CAD build for the part. Positions are in the model's coordinates, mm. Give positions to 0.01 mm unless a question says otherwise; leave off trailing zeros. Loops run counter-clockwise (first coordinate to the right, second up) from the corner with the lowest first, then second, coordinate; pieces in that order, holes last. Notation, with made-up numbers: M 58.25,18.5 L 106.25,18.5 A23 ccw 106.25,36.5 Z; hole C 50,42.5 d7. An arc over 180 degrees is marked long. Answer as CSV lines item,"result".
Autodesk Inventor part; units mm, degrees
ref_plane "YZ Plane" through (0, 0, 0) normal (1, 0, 0) x (0, 1, 0)
ref_plane "XZ Plane" through (0, 0, 0) normal (0, 1, 0) x (-1, 0, 0)
ref_plane "XY Plane" through (0, 0, 0) normal (0, 0, 1) x (1, 0, 0)
sketch "Sketch1" plane through (0, 0, 0) normal (1, 0, 0) x (0, 1, 0)
  line L0 (0, 0) -> (74.6232, 0)
  line L1 (0, 0) -> (85, -6.078)
  line L2 (85, -6.078) -> (0, -6.078)
  line L3 (0, -6.078) -> (0, 0)
  dimension "d0" = 4.09
  dimension "d1" = 85
extrude "Extrusion1" add sketch "Sketch1" along normal blind 75
sketch "Sketch2" plane through (0, 0, -6.078) normal (0, 0, -1) x (-1, 0, 0)
  line L0 (0, 0) -> (0, 85)
  line L1 (0, 85) -> (-75, 85)
  line L2 (-75, 0) -> (-75, 85)
  line L3 (0, 0) -> (-75, 0)
  point P0 (0, 0)
  point P1 (-15, 25)
  point P2 (-60, 60)
  dimension "d4" = 25
  dimension "d5" = 15
  dimension "d6" = 15
  dimension "d7" = 25
hole "Hole1" at (15, 25, -6.078) at (60, 60, -6.078) direction (0, 0, 1) diameter 9 depth 10 tip angle 118
properties part number "skos_smietnik1"
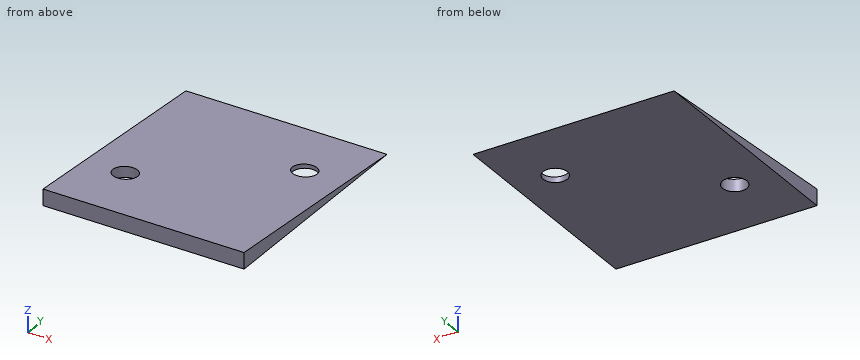
Q1. Wall check: line 1 (X direction, y = 60, z = -5.55); line 2 (X direction, y = 25, z = -4.3); line 3 (Z direction, x = 19.5, y = 21). Give the ranges that are in metal, low to high. Write a range as [from, to].
Solution:
line 1,"x = [0, 55.5], [64.5, 75]"
line 2,"x = [0, 10.5], [19.5, 75]"
line 3,"z = [-6.08, -1.5]"
Q2. Cut at D-D (y = 14). Write the cut outline in (x, z).
Solution:
outline,"M 0,-6.08 L 75,-6.08 L 75,-1 L 0,-1 Z"
Q3. Cut at B-B (y = 25). Write the cut outline in (x, z), and give its area (3 significant figures).
Solution:
outline,"M 0,-6.08 L 10.5,-6.08 L 10.5,-1.79 L 0,-1.79 Z; M 19.5,-6.08 L 75,-6.08 L 75,-1.79 L 19.5,-1.79 Z"
area,"283 mm²"
Q4. Pin check, flat tips, straight feed: P1, Ø5, axis at x = 47, y = 73, coming from the +Z side; P2, Ø10.5, axis at x = 15, y = 25, coming from the +Z side; P3, Ø7, axis at x = 60, y = 60, coming from the -Z side. Stop position of each tip, or through.
Solution:
P1,"stops at z = -5.04"
P2,"stops at z = -1.41"
P3,"passes through"
Q5. Cut at C-C (x = 60). Write the cut outline in (y, z).
Solution:
outline,"M 0,-6.08 L 55.5,-6.08 L 55.5,-3.97 L 0,0 Z; M 64.5,-6.08 L 85,-6.08 L 64.5,-4.61 Z"
Q6. Cut at A-A (x = 13). Write the cut outline in (y, z).
Solution:
outline,"M 0,-6.08 L 20.97,-6.08 L 20.97,-1.5 L 0,0 Z; M 29.03,-6.08 L 85,-6.08 L 29.03,-2.08 Z"
